Geometry check sheet. Reference: the model listing, model coordinates, mm. Face numbers are marked on the shaded views. A direction names the side the tool comes from. Round coordinates to 2 decimals unless told otherwise and drop trailing zeros. Order: outer loops, then holes, each group sorted by start corner. A loop starts at its lowest first (then second) coordinate and runs counter-clockwise, first axis right, second up. Notation, with made-up numbers: (17.25, -25) - (74.25, -25) arc R7 cw to (74.25, -18) - close; hole circle Ø7 at (32.25, 76). An arc over 180 degrees is marked (long way). One line per question, with ' | ' between items. Start each with the question number.
Q1. Sectioned sample at A-A, the plane z = -58. Enter the section's corners in (x, y), then the cut area to 3 significant figures.
Q2. Material ranges on line 1 along X through (y, z) = (61.5, -27); line 2 along Y through (x, z) = (43, -61.5); line 3 along Y through (x, z) = (98, -76), recorded low to high.
Q3. Mould release check, pull along Y, two halves, no side actions. Record for the marked faces 1, 2 and 3: +Y half, -Y half, draft (parallel to the pull), parting line (faces both ways), or undercut.
Q4. Gauge pin test, flat ends, axial feed: P1, Ø1.5, axis at x = 36, y = 6.5, coming from the +Z side; P2, Ø22, axis at x = 78, z = -67, coming from the +Y side; P3, Ø4.5, axis at x = 80.5, y = 62.5, coming from the -Z side; P4, Ø4, axis at x = 104, z = -66.5, coming from the -Y side. Record the tip position at first contact, or that the pin passes through.
Q5. Tool access check on the marked faces 4 and 5. Record the directions out of +Z, -Z, +X, -X, +Y, -Y that give a thin tool (end or side, any length) a straight path to the whole face; none if there is none.
Q6. Sectioned sample at B-B, the plane y = 73.5. Enter the section's corners in (x, z).
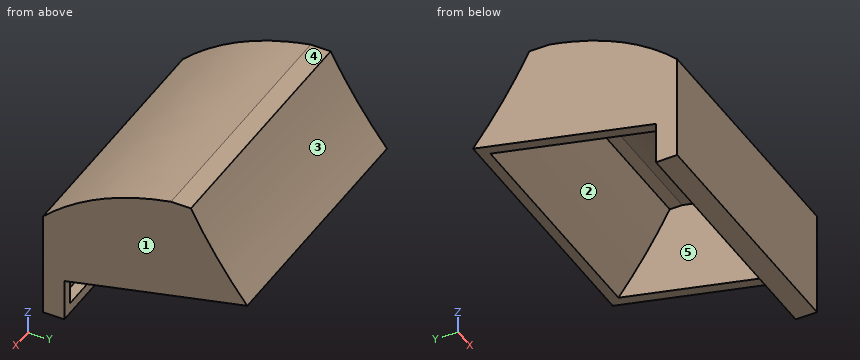
```python
from build123d import *

# Parameters (mm, degrees)
SKETCH1_W           = 120
SKETCH1_H           = 80
BOSS_EXTRUDE1_DEPTH = 100
CUT_EXTRUDE1_DEPTH  = 176.499287748
SKETCH3_R           = 260
CUT_EXTRUDE2_DEPTH  = 176.499287919
SHELL1_T            = -5


with BuildPart() as part:
    # Sketch1 → Boss-Extrude1 (new body)
    with BuildSketch(Plane(origin=(0, 0, 0), x_dir=(1, 0, 0), z_dir=(0, 1, 0))):
        with Locations((60, 40)):
            Rectangle(SKETCH1_W, SKETCH1_H)
    extrude(amount=BOSS_EXTRUDE1_DEPTH)

    # Sketch2 → Cut-Extrude1 (cut, through all)
    with BuildSketch(Plane(origin=(120, 0, 0), x_dir=(0, 0, -1), z_dir=(1, 0, 0))):
        Polygon((80, 10), (60, 10), (40, 100), (80, 100), align=None)
        with BuildLine():
            Line((0, 60), (0, 0))
            Line((0, 0), (30, 0))
            add(Edge.make_bspline(
                [(0, 60), (6.797454451, 24.053758825), (30, 0)],
                knots=[0, 0, 0, 0.927202308, 0.927202308, 0.927202308], degree=2))
        make_face()
    extrude(amount=-CUT_EXTRUDE1_DEPTH, mode=Mode.SUBTRACT)

    # Sketch3 → Cut-Extrude2 (cut, through all)
    with BuildSketch(Plane(origin=(120, 0, 0), x_dir=(0, 0, -1), z_dir=(1, 0, 0))):
        with Locations((-120, 300)):
            Circle(SKETCH3_R)
    extrude(amount=-CUT_EXTRUDE2_DEPTH, mode=Mode.SUBTRACT)

    # Shell1
    shell1_openings = [part.faces().sort_by_distance(p)[0] for p in [
        (60, 10, -70),
        (60, 52.897059769, -50.467320051),
    ]]
    offset(amount=SHELL1_T, openings=shell1_openings, kind=Kind.INTERSECTION)


solid = part.part
```
Determined:
1) outline: (0, 0) - (120, 0) - (120, 19) - (115, 19) - (115, 5) - (5, 5) - (5, 19) - (0, 19) - close | area: 740 mm2
2) line 1: x = 0 to 5, 115 to 120 | line 2: y = 0 to 5 | line 3: y = 0 to 10
3) face 1: draft | face 2: undercut | face 3: +Y half
4) P1: stops at z = -23.6 | P2: stops at y = 10 | P3: stops at z = -5.04 | P4: stops at y = 0
5) face 4: +Z, +X, -X, +Y, -Y | face 5: none
6) outline: (0, -45.89) - (5, -45.89) - (5, -17.56) - (115, -17.56) - (115, -45.89) - (120, -45.89) - (120, -7.66) - (0, -7.66) - close
